```python
from build123d import *

# Parameters (mm, degrees)
SWEEP_THIN1_START              = -85
SWEEP_THIN1_OUTLINE_W          = 10
SWEEP_THIN1_OUTLINE_H          = 26
SWEEP_THIN1_OUTLINE_W_2        = 4
SWEEP_THIN1_OUTLINE_H_2        = 20
SWEEP_THIN1_DEPTH              = 85
BOSS_EXTRUDE1_DEPTH            = 10
CUT_EXTRUDE1_DEPTH             = 1
SKETCH7_R                      = 6
SKETCH7_R_2                    = 4
BOSS_EXTRUDE2_DEPTH            = 1
CUT_EXTRUDE2_REACH             = 101.363
SKETCH8_R                      = 3.991679888
CUT_EXTRUDE2_DIRECTION_2_DEPTH = 100.36297097


# Read off the part's stored shape, not the designer's step: Sweep-Thin1
with BuildPart() as part:
    # Sweep-Thin1 outline → Sweep-Thin1 (new body)
    with BuildSketch(Plane.YZ.offset(SWEEP_THIN1_START)):
        Rectangle(SWEEP_THIN1_OUTLINE_W, SWEEP_THIN1_OUTLINE_H)
        Rectangle(SWEEP_THIN1_OUTLINE_W_2, SWEEP_THIN1_OUTLINE_H_2, mode=Mode.SUBTRACT)
    extrude(amount=SWEEP_THIN1_DEPTH)

    # Sketch5 → Boss-Extrude1 (add)
    with BuildSketch(Plane(origin=(0, 5, 0), x_dir=(1, 0, 0), z_dir=(0, 1, 0))):
        with BuildLine():
            Line((-85, -13), (-85, 13))
            ThreePointArc((-85, 13), (-98, 0), (-85, -13))
        make_face()
    extrude(amount=-BOSS_EXTRUDE1_DEPTH)

    # Sketch6 → Cut-Extrude1 (cut)
    with BuildSketch(Plane(origin=(0, 5, 0), x_dir=(1, 0, 0), z_dir=(0, 1, 0))):
        with BuildLine():
            Line((-89.582575695, 10), (-3, 10))
            Line((-3, 10), (-3, 7.339674458))
            Line((-3, 7.339674458), (-93.193239827, 7.339674458))
            ThreePointArc((-93.193239827, 7.339674458), (-91.524929008, 8.855806086), (-89.582575695, 10))
        make_face()
        with BuildLine():
            Line((-95.246950766, 4), (-3, 4))
            Line((-3, 4), (-3, 1.339674458))
            Line((-3, 1.339674458), (-95.918116703, 1.339674458))
            ThreePointArc((-95.918116703, 1.339674458), (-95.665802982, 2.690844989), (-95.246950766, 4))
        make_face()
        with BuildLine():
            Line((-95.816653826, -2), (-3, -2))
            Line((-3, -2), (-3, -4.660325542))
            Line((-3, -4.660325542), (-94.964003505, -4.660325542))
            ThreePointArc((-94.964003505, -4.660325542), (-95.475125907, -3.357340797), (-95.816653826, -2))
        make_face()
        with BuildLine():
            Line((-92.549834435, -8), (-3, -8))
            Line((-3, -8), (-3, -10.660325542))
            Line((-3, -10.660325542), (-87.712463701, -10.660325542))
            ThreePointArc((-87.712463701, -10.660325542), (-90.300756904, -9.638567126), (-92.549834435, -8))
        make_face()
    cut_extrude1 = extrude(amount=-CUT_EXTRUDE1_DEPTH, mode=Mode.SUBTRACT)

    # Mirror1: Cut-Extrude1 across plane
    add(cut_extrude1.mirror(Plane.ZX), mode=Mode.SUBTRACT)

    # Sketch7 → Boss-Extrude2 (add)
    with BuildSketch(Plane.XZ.offset(5)):
        with Locations((-16, 0)):
            Circle(SKETCH7_R)
        with Locations((-16, 0)):
            Circle(SKETCH7_R_2, mode=Mode.SUBTRACT)
    extrude(amount=-BOSS_EXTRUDE2_DEPTH)

    # Sketch8 → Cut-Extrude2 (cut, up to next)
    with BuildSketch(Plane(origin=(0, -5, 0), x_dir=(-1, 0, 0), z_dir=(0, -1, 0)), mode=Mode.PRIVATE) as cut_extrude2_sk1:
        with Locations(Location((16.005403819, 0.006326373, 0), (0, 0, 270))):
            Circle(SKETCH8_R)
    cut_extrude2_tool1 = extrude(cut_extrude2_sk1.sketch, amount=-CUT_EXTRUDE2_REACH, mode=Mode.PRIVATE) & part.part
    add(cut_extrude2_tool1.solids().sort_by_distance((-16.005404, -5, -0.006326))[0], mode=Mode.SUBTRACT)

    # Sketch8 → Cut-Extrude2 direction 2 (cut)
    with BuildSketch(Plane(origin=(0, -5, 0), x_dir=(-1, 0, 0), z_dir=(0, -1, 0))):
        with Locations(Location((16.005403819, 0.006326373, 0), (0, 0, 270))):
            Circle(SKETCH8_R)
    extrude(amount=CUT_EXTRUDE2_DIRECTION_2_DEPTH, mode=Mode.SUBTRACT)


solid = part.part
```
The listing builds one solid part. Answer for the finished solid, in the listing's coordinates (mm). A direction names the side the tool comes from. Give positions to 0.01 mm unless a question says otherwise; leave off trailing zeros. Order: outer loops, then holes, each group sorted by start corner. A loop starts at its lowest first (then second) coordinate and runs counter-clockwise, first axis right, second up. Notation, with made-up numbers: (64, -23) - (88, -23) arc R19 cw to (88, 4) - close; hole circle Ø4 at (-19.75, -36.5). An arc over 180 degrees is marked (long way). Answer in a Markdown table with one row per item. Add a question column.
Q1. Find the intervals of material crossed by line 1 along Z through (x, y) = (-62.5, 4.75); line 2 along Z through (x, y) = (-34, 1.5); line 3 along Y through (x, z) = (-33, 3.25), in increasing order. Write a range as [from, to].
Q2. Given P1, Ø1.1, axis at y = -4.5, z = -2.5, coming from the -X side; P2, Ø1.3, axis at x = -57, z = 3.5, coming from the -Y side; P3, Ø5, axis at y = 1.5, z = 8, coming from the -X side, each flat-ended and moving along its own axis, determine where each tip first touches the part or whether it passes through.
Q3. The part is cut by section A-A (z = 0). Determine the outline of the cut face in (x, y), then the cut area to 3 significant figures.
Q4. Which of the six approach directions +Z, -Z, +X, -X, +Y, -Y give full straight-line access (tool end or side, diameter ignored) to faces 1 (the flat face through (-47, 4, 9)), 2 (the flat face through (-7, -4, -3)), 3 (the flat face through (-43, 0, -10))?
Q5. For a pull along Y with two mould halves and no side action, classify faces 4 (the flat face through (-43, 2, 0)), 5 (the flat face through (-43, 0, 10)), 6 (the flat face through (-58, -4, -3)), 7 (the flat face through (-47, 4, -9)) as released by +Y, released by -Y, zero draft, split by the parting line, or undercut.
Determined:
| question | item | result |
|---|---|---|
| 1 | line 1 | z = [-13, -10], [-7.34, -4], [-1.34, 2], [4.66, 8], [10.66, 13] |
| 1 | line 2 | z = [-13, -10], [10, 13] |
| 1 | line 3 | y = [-4, -2], [2, 4] |
| 2 | P1 | stops at x = -97.85 |
| 2 | P2 | stops at y = -4 |
| 2 | P3 | stops at x = -96.78 |
| 3 | outline | (-98, -5) - (-20, -5) - (-20, -2) - (-85, -2) - (-85, 2) - (0, 2) - (0, 5) - (-98, 5) - close; (-12.01, -5) - (0, -5) - (0, -2) - (-12.01, -2) - close |
| 3 | area | 616 mm² |
| 4 | face 1 | +Y |
| 4 | face 2 | -Y |
| 4 | face 3 | +X |
| 5 | face 4 | undercut |
| 5 | face 5 | undercut |
| 5 | face 6 | released by -Y |
| 5 | face 7 | released by +Y |
